Build history of the part. All positions in model axes, mm. Face numbers are marked on the shaded views. Coordinates: 2 decimals unless noted, no trailing zeros. Order: outer loops, then holes, each group sorted by start corner. A loop starts at its lowest first (then second) coordinate and runs counter-clockwise, first axis right, second up. Notation, with made-up numbers: (20.25, 22.5) - (67.25, 22.5) arc R9 ccw to (67.25, 39.5) - close; hole circle Ø11 at (-2.5, -11.5). An arc over 180 degrees is marked (long way). Write each question's results on one line, items separated by ' | '.
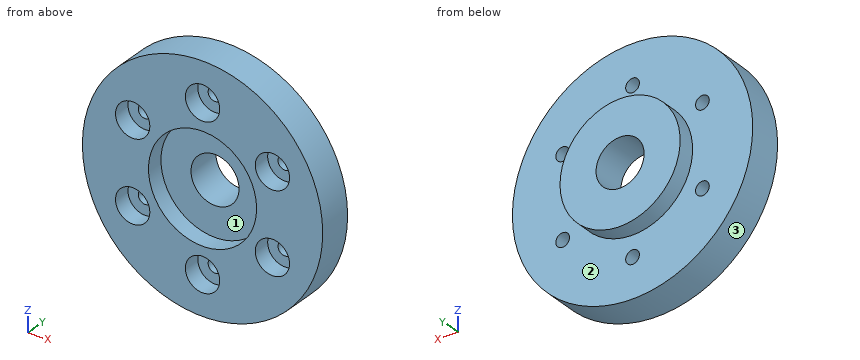
from build123d import *

# Parameters (mm, degrees)
SKETCH1_R           = 35
BOSS_EXTRUDE1_DEPTH = 15
SKETCH3_R           = 15.75
CUT_EXTRUDE1_DEPTH  = 5
SKETCH4_R           = 7
CUT_EXTRUDE2_DEPTH  = 11
SKETCH5_R           = 35
SKETCH5_R_2         = 17.5
CUT_EXTRUDE3_DEPTH  = 5
SKETCH6_R           = 2
CUT_EXTRUDE4_DEPTH  = 11
SKETCH7_R           = 5
SKETCH7_R_2         = 2
CUT_EXTRUDE5_DEPTH  = 5


with BuildPart() as part:
    # Sketch1 → Boss-Extrude1 (new body)
    with BuildSketch(Plane(origin=(0, 0, 0), x_dir=(1, 0, 0), z_dir=(0, 1, 0))):
        Circle(SKETCH1_R)
    extrude(amount=BOSS_EXTRUDE1_DEPTH)

    # Sketch3 → Cut-Extrude1 (cut)
    with BuildSketch(Plane.XZ):
        Circle(SKETCH3_R)
    extrude(amount=-CUT_EXTRUDE1_DEPTH, mode=Mode.SUBTRACT)

    # Sketch4 → Cut-Extrude2 (cut, through all)
    with BuildSketch(Plane.XZ.offset(-5)):
        Circle(SKETCH4_R)
    extrude(amount=-CUT_EXTRUDE2_DEPTH, mode=Mode.SUBTRACT)

    # Sketch5 → Cut-Extrude3 (cut)
    with BuildSketch(Plane(origin=(0, 15, 0), x_dir=(1, 0, 0), z_dir=(0, 1, 0))):
        Circle(SKETCH5_R)
        Circle(SKETCH5_R_2, mode=Mode.SUBTRACT)
    extrude(amount=-CUT_EXTRUDE3_DEPTH, mode=Mode.SUBTRACT)

    # Sketch6 → Cut-Extrude4 (cut, through all)
    with BuildSketch(Plane(origin=(0, 10, 0), x_dir=(1, 0, 0), z_dir=(0, 1, 0))):
        with Locations((0, 23.5)):
            Circle(SKETCH6_R)
        with Locations((20.351596989, 11.75)):
            Circle(SKETCH6_R)
        with Locations((20.351596989, -11.75)):
            Circle(SKETCH6_R)
        with Locations((0, -23.5)):
            Circle(SKETCH6_R)
        with Locations((-20.351596989, -11.75)):
            Circle(SKETCH6_R)
        with Locations((-20.351596989, 11.75)):
            Circle(SKETCH6_R)
    extrude(amount=-CUT_EXTRUDE4_DEPTH, mode=Mode.SUBTRACT)

    # Sketch7 → Cut-Extrude5 (cut)
    with BuildSketch(Plane.XZ):
        with Locations((0, 23.5)):
            Circle(SKETCH7_R)
        with Locations((0, 23.5)):
            Circle(SKETCH7_R_2, mode=Mode.SUBTRACT)
        with Locations((20.351596989, 11.75)):
            Circle(SKETCH7_R)
        with Locations((20.351596989, 11.75)):
            Circle(SKETCH7_R_2, mode=Mode.SUBTRACT)
        with Locations((20.351596989, -11.75)):
            Circle(SKETCH7_R)
        with Locations((20.351596989, -11.75)):
            Circle(SKETCH7_R_2, mode=Mode.SUBTRACT)
        with Locations((0, -23.5)):
            Circle(SKETCH7_R)
        with Locations((0, -23.5)):
            Circle(SKETCH7_R_2, mode=Mode.SUBTRACT)
        with Locations((-20.351596989, -11.75)):
            Circle(SKETCH7_R)
        with Locations((-20.351596989, -11.75)):
            Circle(SKETCH7_R_2, mode=Mode.SUBTRACT)
        with Locations((-20.351596989, 11.75)):
            Circle(SKETCH7_R)
        with Locations((-20.351596989, 11.75)):
            Circle(SKETCH7_R_2, mode=Mode.SUBTRACT)
    extrude(amount=-CUT_EXTRUDE5_DEPTH, mode=Mode.SUBTRACT)


solid = part.part
1. Drop flat-ended pins along their axis: pin 1 Ø6 at (x, y) = (-14, 13.5) entering from +Z; pin 2 Ø8 at (x, z) = (0.5, 23.5) entering from -Y; pin 3 Ø1.5 at (x, y) = (-8.5, 3) entering from -Z. Give the stop position or say it passes through.
Solved:
pin 1: stops at z = 13.61 | pin 2: stops at y = 5 | pin 3: stops at z = -34.13
2. Band-saw the part on D-D on x = 21. Give the cut face in (y, z).
Solved:
outline: (0, -28) - (10, -28) - (10, -13.64) - (5, -13.64) - (5, -16.71) - (0, -16.71) - close; (0, -6.79) - (5, -6.79) - (5, -9.86) - (10, -9.86) - (10, 9.86) - (5, 9.86) - (5, 6.79) - (0, 6.79) - close; (0, 16.71) - (5, 16.71) - (5, 13.64) - (10, 13.64) - (10, 28) - (0, 28) - close
3. Two-plate mould, pull along X, no slides. Class the marked faces 1, 2 and 3: +X half, -X half, draft (parallel to the pull), parting line (faces both ways), or undercut.
Solved:
face 1: undercut | face 2: draft | face 3: parting line
4. Band-saw the part on C-C on z = 0. Give the cut face in (x, y).
Solved:
outline: (-35, 0) - (-15.75, 0) - (-15.75, 5) - (-7, 5) - (-7, 15) - (-17.5, 15) - (-17.5, 10) - (-35, 10) - close; (7, 5) - (15.75, 5) - (15.75, 0) - (35, 0) - (35, 10) - (17.5, 10) - (17.5, 15) - (7, 15) - close
5. Probe line 1 (Z direction, x = 0, y = 2.65); line 2 (Z direction, x = 20.5, y = 8); line 3 (Z direction, x = 19, y = 1). List the from-to ranges inside material, lowest first.
Solved:
line 1: z = -35 to -28.5, -18.5 to -15.75, 15.75 to 18.5, 28.5 to 35 | line 2: z = -28.37 to -13.74, -9.76 to 9.76, 13.74 to 28.37 | line 3: z = -29.39 to -16.56, -6.94 to 6.94, 16.56 to 29.39
6. Band-saw the part on B-B on y = 7.25. Give the cut face in (x, z), then the cut area to 3 significant figures.
Solved:
outline: circle Ø70 at (0, 0); hole circle Ø4 at (-20.35, -11.75); hole circle Ø4 at (-20.35, 11.75); hole circle Ø14 at (0, 0); hole circle Ø4 at (0, -23.5); hole circle Ø4 at (0, 23.5); hole circle Ø4 at (20.35, -11.75); hole circle Ø4 at (20.35, 11.75) | area: 3,620 mm2
7. Band-saw the part on A-A on x = 0. Give the number of separate pieces and of enclosed holes in the cut face, then the cut area to 4 significant figures.
Solved:
separate pieces: 4 | enclosed holes: 0 | area: 437.5 mm2
